from build123d import *

# Parameters (mm, degrees)
SKETCH_1_W          = 483
SKETCH_1_H          = 305
EXTRUDE_1_DEPTH     = 30
SKETCH_2_W          = 443
SKETCH_2_H          = 265
EXTRUDE_2_DEPTH     = 140
FILLET_2_R          = 20
CUT_EXTRUDE_START   = -20
CUT_EXTRUDE_3_DEPTH = 576.998322145
SKETCH_7_R          = 42.5
SKETCH_7_R_2        = 29.5
EXTRUDE_3_DEPTH     = 50
SKETCH_7_5_R        = 42.5
SKETCH_7_5_R_2      = 29.5
CUT_EXTRUDE_5_DEPTH = 20
SKETCH_7_6_R        = 29.5
CUT_EXTRUDE_6_DEPTH = 40
SKETCH_9_R          = 17.8766886
EXTRUDE_4_DEPTH     = 20


with BuildPart() as part:
    # 草图1 → 凸台-拉伸1 (new body)
    with BuildSketch(Plane(origin=(0, 0, 0), x_dir=(1, 0, 0), z_dir=(0, 1, 0))):
        with Locations((-241.5, 152.5)):
            Rectangle(SKETCH_1_W, SKETCH_1_H)
    extrude(amount=EXTRUDE_1_DEPTH)

    # 草图2 → 凸台-拉伸2 (add)
    with BuildSketch(Plane(origin=(0, 30, 0), x_dir=(1, 0, 0), z_dir=(0, 1, 0))):
        with Locations((-241.5, 152.5)):
            Rectangle(SKETCH_2_W, SKETCH_2_H)
    extrude(amount=EXTRUDE_2_DEPTH)

    # 圆角2
    fillet_2_edges = [part.edges().sort_by_distance(p)[0] for p in [
        (-463, 100, -285),
        (-463, 100, -20),
        (-20, 100, -20),
        (-20, 100, -285),
        (0, 15, 0),
        (-483, 15, 0),
        (-483, 15, -305),
        (0, 15, -305),
    ]]
    fillet(fillet_2_edges, radius=FILLET_2_R)

    # 草图5 → 切除-拉伸3 (cut, through all)
    with BuildSketch(Plane(origin=(0, 170, 0), x_dir=(1, 0, 0), z_dir=(0, 1, 0)).offset(CUT_EXTRUDE_START)):
        with BuildLine():
            Line((-40, 60), (-40, 245))
            ThreePointArc((-40, 245), (-45.857864376, 259.142135624), (-60, 265))
            Line((-60, 265), (-423, 265))
            ThreePointArc((-423, 265), (-437.142135624, 259.142135624), (-443, 245))
            Line((-443, 245), (-443, 60))
            ThreePointArc((-443, 60), (-437.142135624, 45.857864376), (-423, 40))
            Line((-423, 40), (-60, 40))
            ThreePointArc((-60, 40), (-45.857864376, 45.857864376), (-40, 60))
        make_face()
    extrude(amount=-CUT_EXTRUDE_3_DEPTH, mode=Mode.SUBTRACT)

    # 草图7 → 凸台-拉伸3 (add)
    # profile 1 of 2: a face of its own
    with BuildSketch(Plane(origin=(0, 170, 0), x_dir=(1, 0, 0), z_dir=(0, 1, 0))):
        with BuildLine():
            Line((-368, 207.5), (-463, 207.5))
            Line((-463, 207.5), (-463, 97.5))
            Line((-463, 97.5), (-368, 97.5))
            ThreePointArc((-368, 97.5), (-313, 152.5), (-368, 207.5))
        make_face()
        with Locations((-368, 152.5)):
            Circle(SKETCH_7_R, mode=Mode.SUBTRACT)
    # profile 2 of 2: a face of its own
    with BuildSketch(Plane(origin=(0, 170, 0), x_dir=(1, 0, 0), z_dir=(0, 1, 0))):
        with Locations((-368, 152.5)):
            Circle(SKETCH_7_R)
        with Locations(Location((-368, 152.5, 0), (0, 0, 270))):
            Circle(SKETCH_7_R_2, mode=Mode.SUBTRACT)
    extrude(amount=-EXTRUDE_3_DEPTH)

    # 草图7<5> → 切除-拉伸5 (cut)
    with BuildSketch(Plane(origin=(0, 170, 0), x_dir=(1, 0, 0), z_dir=(0, 1, 0))):
        with Locations(Location((-368, 152.5, 0), (0, 0, 270))):
            Circle(SKETCH_7_5_R)
        with Locations(Location((-368, 152.5, 0), (0, 0, 270))):
            Circle(SKETCH_7_5_R_2, mode=Mode.SUBTRACT)
    extrude(amount=-CUT_EXTRUDE_5_DEPTH, mode=Mode.SUBTRACT)


with BuildPart() as cut_extrude_5_piece_1:
    # of the separate pieces the step leaves, piece 1, a body of its own (cut_extrude_5_pieces)
    add(part.part.solids().sort_by_distance((-20, 0, 0))[0])

    # 草图9 → 凸台-拉伸4 (add)
    with BuildSketch(Plane.XY.offset(-20)):
        with BuildLine():
            Line((-87.75, 30), (-87.75, 85))
            ThreePointArc((-87.75, 85), (-130.75, 128), (-173.75, 85))
            Line((-173.75, 85), (-173.75, 30))
            Line((-173.75, 30), (-87.75, 30))
        make_face()
        with Locations(Location((-130.75, 85, 0), (0, 0, 180))):
            Circle(SKETCH_9_R, mode=Mode.SUBTRACT)
    extrude(amount=EXTRUDE_4_DEPTH)


with BuildPart() as cut_extrude_5_piece_2:
    # of the separate pieces the step leaves, piece 2, a body of its own (cut_extrude_5_pieces)
    add(part.part.solids().sort_by_distance((-368, 170, -123))[0])

    # 草图7<6> → 切除-拉伸6 (cut)
    with BuildSketch(Plane(origin=(0, 170, 0), x_dir=(1, 0, 0), z_dir=(0, 1, 0))):
        with Locations(Location((-368, 152.5, 0), (0, 0, 270))):
            Circle(SKETCH_7_6_R)
    extrude(amount=-CUT_EXTRUDE_6_DEPTH, mode=Mode.SUBTRACT)


solid = cut_extrude_5_piece_1.part
Could you check a few things on this model? Use its own coordinates, in mm. A direction names the side the tool comes from. Round coordinates to 2 decimals unless told otherwise and drop trailing zeros. Loops run counter-clockwise (first coordinate to the right, second up) from the corner with the lowest first, then second, coordinate; pieces in that order, holes last. Notation, with made-up numbers: (38.25, 47) -> (75.25, 47) arc R5 ccw to (75.25, 53) -> close; hole circle Ø9 at (43.25, 47.5). An arc over 180 degrees is marked (long way). Use CSV: the item, a comma, the result in double quotes.
(1) Suppose I cut it at B-B on y = 61.5. Write out the boundary of the cut face in (x, z), plus the area to 3 significant figures.
Return value:
outline,"(-463, -265) arc R20 ccw to (-443, -285) -> (-40, -285) arc R20 ccw to (-20, -265) -> (-20, -40) arc R20 ccw to (-40, -20) -> (-87.75, -20) -> (-87.75, 0) -> (-173.75, 0) -> (-173.75, -20) -> (-443, -20) arc R20 ccw to (-463, -40) -> close; hole (-443, -245) arc R20 ccw to (-423, -265) -> (-60, -265) arc R20 ccw to (-40, -245) -> (-40, -60) arc R20 ccw to (-60, -40) -> (-423, -40) arc R20 ccw to (-443, -60) -> close"
area,"28,400 mm²"
(2) For faces 5 (the cylindrical face through (-45.703, 76.05, -258.986)), 6 (the flat face through (-377, 150, -181)), 7 (the cylindrical face through (-26.014, 100.98, -25.703)), 8 (the cylindrical face through (-25.703, 100.98, -278.986)), 9 (the flat face through (-244, 99, -285)), which set-ups out of +Z, -Z, +X, -X, +Y, -Y let a thin tool reach every point of the face, with its end or its side?
Return value:
face 5,"-Y"
face 6,"+Y"
face 7,"+Z, +X, +Y"
face 8,"-Z, +X, +Y"
face 9,"-Z, +X, -X, +Y"
(3) Suppose I cut it at D-D on x = -296. Write out the boundary of the cut face in (y, z).
Return value:
outline,"(0, -305) -> (30, -305) -> (30, -285) -> (170, -285) -> (170, -20) -> (30, -20) -> (30, 0) -> (0, 0) -> (0, -40) -> (150, -40) -> (150, -265) -> (0, -265) -> close"
(4) Suppose I cut it at A-A on z = -152.5. Write out the boundary of the cut face in (x, y), plus the area to 3 significant figures.
Return value:
outline,"(-483, 0) -> (-443, 0) -> (-443, 120) -> (-397.5, 120) -> (-397.5, 150) -> (-410.5, 150) -> (-410.5, 170) -> (-463, 170) -> (-463, 30) -> (-483, 30) -> close; (-338.5, 120) -> (-313, 120) -> (-313, 150) -> (-40, 150) -> (-40, 0) -> (0, 0) -> (0, 30) -> (-20, 30) -> (-20, 170) -> (-325.5, 170) -> (-325.5, 150) -> (-338.5, 150) -> close"
area,"16,500 mm²"
(5) Suppose I cut it at C-C on x = -375. Write out the boundary of the cut face in (y, z), plus the area to 3 significant figures.
Return value:
outline,"(0, -305) -> (30, -305) -> (30, -285) -> (170, -285) -> (170, -194.42) -> (150, -194.42) -> (150, -181.16) -> (120, -181.16) -> (120, -207.5) -> (150, -207.5) -> (150, -265) -> (0, -265) -> close; (0, -40) -> (150, -40) -> (150, -97.5) -> (120, -97.5) -> (120, -123.84) -> (150, -123.84) -> (150, -110.58) -> (170, -110.58) -> (170, -20) -> (30, -20) -> (30, 0) -> (0, 0) -> close"
area,"12,400 mm²"
(6) Will these pins go through, and if not, where does the flat tip stop? pin 1 Ø16 at (y, z) = (49, -7) entering from +X; pin 2 Ø6 at (y, z) = (66, -9.5) entering from -X; pin 3 Ø4 at (y, z) = (105, -54) entering from +X.
Return value:
pin 1,"stops at x = -87.75"
pin 2,"stops at x = -173.75"
pin 3,"stops at x = -20"
(7) If I drill on probe 1 along Y at (x, z) = (-130.75, -13); probe 2 along X at (y, z) = (133, -152); probe 3 along X at (y, z) = (136, -210), over which ranges is the centre line in solid material (lowest first)? Write a range as [from, to].
Return value:
probe 1,"y = [0, 67.12], [102.88, 128]"
probe 2,"x = [-463, -397.5], [-338.5, -313], [-40, -20]"
probe 3,"x = [-463, -443], [-40, -20]"
(8) If we mould it in two halves opening along X, with no side actions, what happens to faces 1 (the flat face through (-244, 76, -40)), 2 (the flat face through (-245, 15, -305)), 3 (the flat face through (-239, 76, -265)), 4 (the flat face through (-483, 15, -151))? For each: +X half, -X half, draft (parallel to the pull), parting line (faces both ways), or undercut.
Return value:
face 1,"undercut"
face 2,"draft"
face 3,"undercut"
face 4,"-X half"
